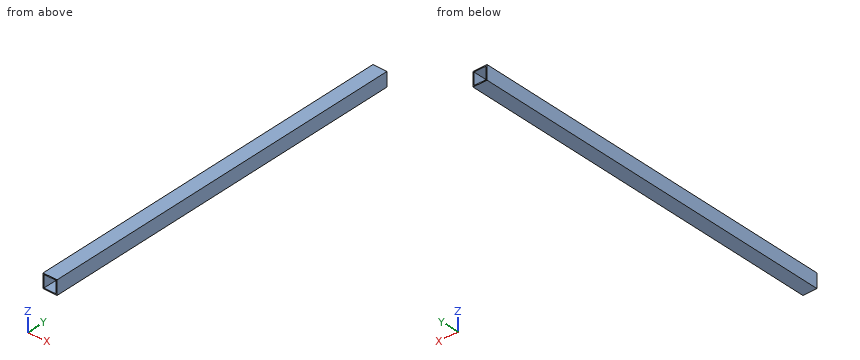
```python
from build123d import *

# Parameters (mm, degrees)
SKETCH_W   = 30
SKETCH_H   = 30
SKETCH_W_2 = 26
SKETCH_H_2 = 26
PAD_DEPTH  = 800


with BuildPart() as part:
    # Sketch → Pad (new body)
    with BuildSketch(Plane.XZ):
        with Locations((15, 15)):
            Rectangle(SKETCH_W, SKETCH_H)
        with Locations((15, 15)):
            Rectangle(SKETCH_W_2, SKETCH_H_2, mode=Mode.SUBTRACT)
    extrude(amount=PAD_DEPTH)


solid = part.part
```
Part model, mm, in its own coordinate system. Round coordinates to 2 decimals unless told otherwise and drop trailing zeros. Loops run counter-clockwise (first coordinate to the right, second up) from the corner with the lowest first, then second, coordinate; pieces in that order, holes last.
1. Slice it at B-B (x = 19.75). Give the cut face in (y, z).
Solutions:
outline: (-800, 0) - (0, 0) - (0, 2) - (-800, 2) - close; (-800, 28) - (0, 28) - (0, 30) - (-800, 30) - close
2. Flat gauge pins, fed straight in: pin 1 (1.5 mm diameter, centred on y = -172.5, z = 4.5, fed in from -X); pin 2 (10 mm diameter, centred on x = 9.5, z = 22, fed in from -Y) (3 decimals). Where does each tip first touch, or does it go through?
Solutions:
pin 1: stops at x = 0
pin 2: passes through
3. Slice it at A-A (z = 20.75). Give the cut face in (x, y).
Solutions:
outline: (0, -800) - (2, -800) - (2, 0) - (0, 0) - close; (28, -800) - (30, -800) - (30, 0) - (28, 0) - close
4. Slice it at C-C (y = -94.5). Give the cut face in (x, z), and give its area (3 significant figures).
Solutions:
outline: (0, 0) - (30, 0) - (30, 30) - (0, 30) - close; hole (2, 2) - (28, 2) - (28, 28) - (2, 28) - close
area: 224 mm2
5. Drill centre line: line 1 along X through (y, z) = (-315.5, 10). Where is it in solid material? Low to high.
Solutions:
line 1: x = 0 to 2, 28 to 30
